Can you work these out from the model? Positions are in its coordinate system, mm. Face numbers are marked on the shaded views. Coordinates: 2 decimals unless noted, no trailing zeros. Loops run counter-clockwise (first coordinate to the right, second up) from the corner with the lowest first, then second, coordinate; pieces in that order, holes last. Notation, with made-up numbers: M -26,-14 L 29,-14 A29 cw 29,13 Z; hole C -23.75,26 d4. An arc over 180 degrees is marked long. Return JSON: item names as keys, results as strings. Group by question number.
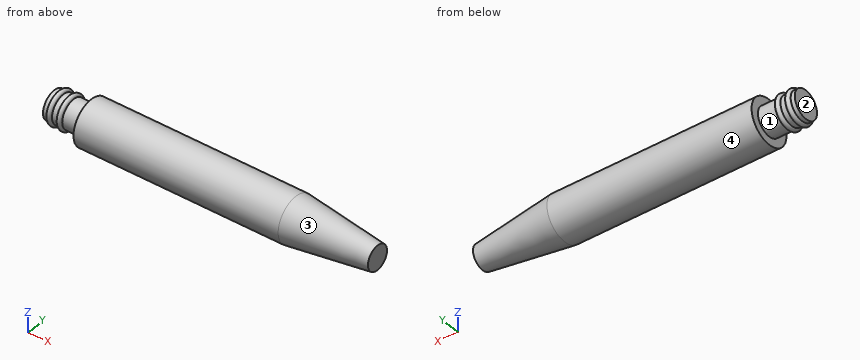
```python
from build123d import *


with BuildPart() as part:
    # Sketch1 → Revolve1 (revolve)
    with BuildSketch(Plane.XY, mode=Mode.PRIVATE) as revolve1_sk:
        with BuildLine():
            Line((172.16927252, 153.812567331), (192.23527252, 153.812567331))
            Line((192.23527252, 153.812567331), (192.23527252, 154.574567331))
            Line((192.23527252, 154.574567331), (187.15527252, 155.209567331))
            Line((187.15527252, 155.209567331), (174.45527252, 155.209567331))
            Line((174.45527252, 155.209567331), (174.45527252, 154.701567331))
            Line((174.45527252, 154.701567331), (173.36307252, 154.701567331))
            ThreePointArc((173.36307252, 154.701567331), (173.21067252, 154.853967331), (173.05827252, 154.701567331))
            Line((173.05827252, 154.701567331), (172.72807252, 154.701567331))
            ThreePointArc((172.72807252, 154.701567331), (172.57567252, 154.853967331), (172.42327252, 154.701567331))
            Line((172.42327252, 154.701567331), (172.16927252, 154.701567331))
            Line((172.16927252, 154.701567331), (172.16927252, 153.812567331))
        make_face()
    revolve(revolve1_sk.sketch.rotate(Axis((172.16927252, 153.812567331, 0), (1, 0, 0)), 90), axis=Axis((172.16927252, 153.812567331, 0), (1, 0, 0)))


solid = part.part
```
1) If I drill on line 1 (Y direction, x = 187.75, z = 1.05); line 2 (Z direction, x = 176.75, y = 153.7); line 3 (Z direction, x = 190.75, y = 154.1), over which ranges is the centre line in solid material (lowest first)? Write a range as from..to.
2) If we mould it in two halves opening along X, with no side actions, what happens to the marked faces 1, 2, 3 and 4? For each: +X half, -X half, draft (parallel to the pull), parting line (faces both ways), or undercut.
3) For pin 1 (1.5 mm diameter, centred on x = 185.5, z = -0.5, fed in from +Y), with a flat end and sliding along its axis, tell me the tip position at first contact or that it passes through.
4) Suppose I cut it at C-C, the plane x = 189. List the corners of the cut face in (y, z) for me, then the cut area to 3 significant figures.
5) Suppose I cut it at A-A, the plane z = 0. List the corners of the cut face in (x, y) for me, then the cut area to 3 significant figures.
6) Suppose I cut it at B-B, the plane x = 181. List the corners of the cut face in (y, z) for me, then the cut area to 3 significant figures.
Returned:
{
 "1": {"line 1": "y = 153.01..154.62", "line 2": "z = -1.39..1.39", "line 3": "z = -0.9..0.9"},
 "2": {"face 1": "undercut", "face 2": "-X half", "face 3": "+X half", "face 4": "draft"},
 "3": {"pin 1": "stops at y = 155.21"},
 "4": {"outline": "C 153.81,0 d2.33", "area": "4.27 mm²"},
 "5": {"outline": "M 172.17,152.92 L 172.42,152.92 A0.15 ccw 172.73,152.92 L 173.06,152.92 A0.15 ccw 173.36,152.92 L 174.46,152.92 L 174.46,152.42 L 187.16,152.42 L 192.24,153.05 L 192.24,154.57 L 187.16,155.21 L 174.46,155.21 L 174.46,154.7 L 173.36,154.7 A0.15 ccw 173.06,154.7 L 172.73,154.7 A0.15 ccw 172.42,154.7 L 172.17,154.7 Z", "area": "50.7 mm²"},
 "6": {"outline": "C 153.81,0 d2.79", "area": "6.13 mm²"}
}
